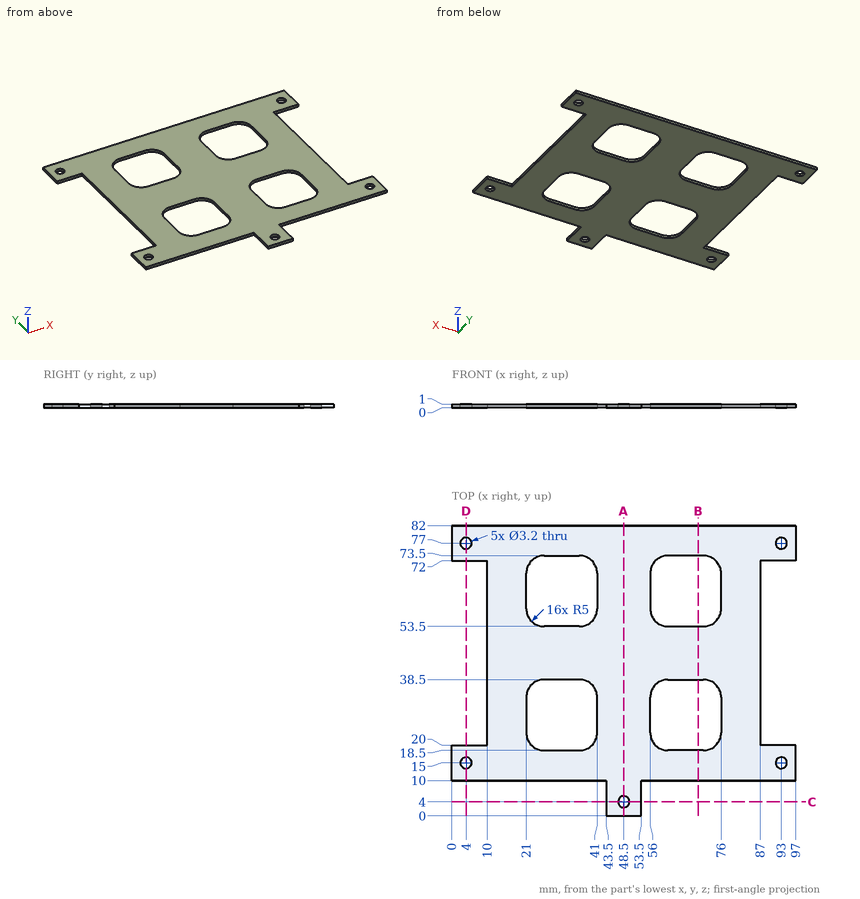
Drawing for the job (mm, zero at the part's lowest x, y, z). Give positions to 0.01 mm unless a question says otherwise; leave off trailing zeros. Loops run counter-clockwise (first coordinate to the right, second up) from the corner with the lowest first, then second, coordinate; pieces in that order, holes last.
(1) Pin check, flat tips, straight feed: pin 1 (3 mm diameter, centred on x = 48.5, y = 4, fed in from -Z); pin 2 (0.5 mm diameter, centred on x = 11, z = 0.5, fed in from -Y); pin 3 (0.5 mm diameter, centred on y = 36.5, z = 0.5, fed in from -X). Stop position of each tip, or through.
Return value:
pin 1: passes through
pin 2: stops at y = 10
pin 3: stops at x = 10
(2) Band-saw the part on B-B (x = 69.5). Write the cut outline in (y, z), and give its area (3 significant figures).
Return value:
outline: (10, 0) - (18.5, 0) - (18.5, 1) - (10, 1) - close; (38.5, 0) - (53.5, 0) - (53.5, 1) - (38.5, 1) - close; (73.5, 0) - (82, 0) - (82, 1) - (73.5, 1) - close
area: 32.0 mm2
(3) Drill centre lines: line 1 along Y through (x, z) = (4, 0.45); line 2 along X through (y, z) = (30, 0.65); line 3 along Y through (x, z) = (25.5, 0.6). Where is each one in solid material? Low to high.
Return value:
line 1: y = 10 to 13.4, 16.6 to 20, 72 to 75.4, 78.6 to 82
line 2: x = 10 to 21, 41 to 56, 76 to 87
line 3: y = 10 to 18.53, 38.47 to 53.53, 73.47 to 82
(4) Band-saw the part on D-D (x = 4). Write the cut outline in (y, z), and give its area (3 significant figures).
Return value:
outline: (10, 0) - (13.4, 0) - (13.4, 1) - (10, 1) - close; (16.6, 0) - (20, 0) - (20, 1) - (16.6, 1) - close; (72, 0) - (75.4, 0) - (75.4, 1) - (72, 1) - close; (78.6, 0) - (82, 0) - (82, 1) - (78.6, 1) - close
area: 13.6 mm2
(5) Band-saw the part on A-A (x = 48.5). Write the cut outline in (y, z).
Return value:
outline: (0, 0) - (2.4, 0) - (2.4, 1) - (0, 1) - close; (5.6, 0) - (82, 0) - (82, 1) - (5.6, 1) - close
(6) Band-saw the part on C-C (y = 4). Write the cut outline in (x, z), and give its area (3 significant figures).
Return value:
outline: (43.5, 0) - (46.9, 0) - (46.9, 1) - (43.5, 1) - close; (50.1, 0) - (53.5, 0) - (53.5, 1) - (50.1, 1) - close
area: 6.80 mm2
